The listing builds one solid part. Answer for the finished solid, in the listing's coordinates (mm). Face numbers are marked on the shaded views. A direction names the side the tool comes from. Give positions to 0.01 mm unless a question says otherwise; leave off trailing zeros. Loops run counter-clockwise (first coordinate to the right, second up) from the corner with the lowest first, then second, coordinate; pieces in that order, holes last. Notation, with made-up numbers: M -25.5,61.5 L -20.5,61.5 A16 ccw -20.5,69.5 Z; hole C -10,82.5 d3. An arc over 180 degrees is marked long. Return JSON: item names as keys, results as strings.
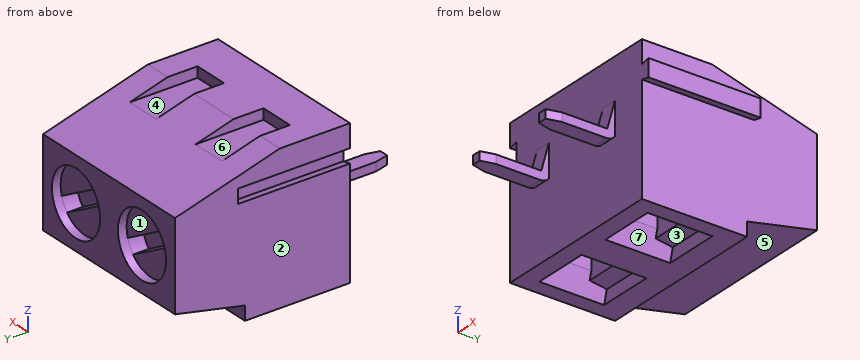
from build123d import *
from build123d.topology import SkipClean

# Parameters (mm, degrees)
BOSS_EXTRUDE1_DEPTH = 2.5
CUT_EXTRUDE1_DEPTH  = 1.25
CHAMFER1_SIZE       = 0.35
CHAMFER1_SIZE_2     = 1.3
CUT_EXTRUDE2_DEPTH  = 1
SKETCH5_R           = 1.825
CUT_EXTRUDE3_DEPTH  = 0.5
CUT_EXTRUDE4_DEPTH  = 0.9
BOSS_EXTRUDE3_DEPTH = 0.45
CHAMFER2_SIZE       = 0.2
CHAMFER2_SIZE2      = 0.79
MIRROR1_START       = -1.36978926
MIRROR1_OUTLINE_W   = 4
MIRROR1_OUTLINE_H   = 0.498489558
MIRROR1_DEPTH       = 0.193883275
LPATTERN1_COUNT     = 2
LPATTERN1_PITCH     = 5
BOSS_EXTRUDE2_DEPTH = 6.4
CUT_EXTRUDE5_DEPTH  = 6.4


# Read off the part's stored shape, not the designer's step: Mirror1
with BuildPart() as part:
    # Sketch2 → Boss-Extrude1 (new, symmetric)
    with BuildSketch(Plane(origin=(0, 0, 0), x_dir=(0, 0, -1), z_dir=(1, 0, 0))):
        Polygon((-4.15, 4), (-4.15, 0), (4.15, 0), (4.15, 6), (3.35, 6), (2.5, 9.99), (-2.5, 9.99), align=None)
    extrude(amount=BOSS_EXTRUDE1_DEPTH, both=True)

    # Sketch3 → Cut-Extrude1 (cut, symmetric)
    with BuildSketch(Plane(origin=(0, 0, 0), x_dir=(0, 0, -1), z_dir=(1, 0, 0))):
        Polygon((4.15, 1), (2.58, 1.84), (-2.25, 1.84), (-2.25, 3.7), (3.2988, 3.7), (3.4175, 4.7), (4.15, 4.7), align=None)
    extrude(amount=CUT_EXTRUDE1_DEPTH, both=True, mode=Mode.SUBTRACT)

    # Chamfer1
    # the kernel refuses this chamfer: 1.3, 0.35 mm, written as the material it takes off along each edge
    with BuildSketch(Plane(origin=(1.25, 4.7, -4.15), x_dir=(0.9905947308102195, 0, -0.1368286493795385), z_dir=(0, -1, 0))) as chamfer1_piece_1_section:
        Polygon((CHAMFER1_SIZE * 0.99059473081, CHAMFER1_SIZE * 0.13682864938), (-CHAMFER1_SIZE_2 * 0.13682864938, CHAMFER1_SIZE_2 * 0.99059473081), (0, 0), align=None)
    chamfer1_piece_1 = extrude(amount=7.075699234, mode=Mode.PRIVATE)
    chamfer1_piece_1 = split(chamfer1_piece_1, bisect_by=Plane(origin=(1.398374335, 1.802145787, -2.650751327), z_dir=(0, 0.8817303170442501, -0.47175380020201896)), keep=Keep.TOP, mode=Mode.PRIVATE)
    chamfer1_piece_1 = split(chamfer1_piece_1, bisect_by=Plane(origin=(1.398374335, 4.303686728, -3.370457615), z_dir=(0, -0.11787251100077023, -0.9930287363165143)), keep=Keep.TOP, mode=Mode.PRIVATE)
    add(chamfer1_piece_1, mode=Mode.SUBTRACT)
    with BuildSketch(Plane(origin=(1.25, 8.075699234, -4.15), x_dir=(0.9905947308102195, 0, -0.1368286493795385), z_dir=(0, -1, 0))) as chamfer1_piece_2_section:
        Polygon((CHAMFER1_SIZE * 0.99059473081, CHAMFER1_SIZE * 0.13682864938), (-CHAMFER1_SIZE_2 * 0.13682864938, CHAMFER1_SIZE_2 * 0.99059473081), (0, 0), align=None)
    chamfer1_piece_2 = extrude(amount=10.451398467, mode=Mode.PRIVATE)
    chamfer1_piece_2 = split(chamfer1_piece_2, bisect_by=Plane(origin=(1.281910217, 1.867643019, -2.528333882), z_dir=(0, 0.8817303170442501, -0.47175380020201896)), keep=Keep.TOP, mode=Mode.PRIVATE)
    chamfer1_piece_2 = split(chamfer1_piece_2, bisect_by=Plane(origin=(1.281910217, 3.7, -3.087047323), z_dir=(0, -1, 0)), keep=Keep.TOP, mode=Mode.PRIVATE)
    add(chamfer1_piece_2, mode=Mode.SUBTRACT)
    with BuildSketch(Plane(origin=(-1.25, 4.7, -4.15), x_dir=(-0.9905947308102195, 0, -0.1368286493795385), z_dir=(0, -1, 0))) as chamfer1_piece_3_section:
        Polygon((CHAMFER1_SIZE * 0.99059473081, -CHAMFER1_SIZE * 0.13682864938), (-CHAMFER1_SIZE_2 * 0.13682864938, -CHAMFER1_SIZE_2 * 0.99059473081), (0, 0), align=None)
    chamfer1_piece_3 = extrude(amount=7.075699234, mode=Mode.PRIVATE)
    chamfer1_piece_3 = split(chamfer1_piece_3, bisect_by=Plane(origin=(-1.398374335, 1.802145787, -2.650751327), z_dir=(0, 0.8817303170442501, -0.47175380020201896)), keep=Keep.TOP, mode=Mode.PRIVATE)
    chamfer1_piece_3 = split(chamfer1_piece_3, bisect_by=Plane(origin=(-1.398374335, 4.303686728, -3.370457615), z_dir=(0, -0.11787251100077023, -0.9930287363165143)), keep=Keep.TOP, mode=Mode.PRIVATE)
    add(chamfer1_piece_3, mode=Mode.SUBTRACT)
    with BuildSketch(Plane(origin=(-1.25, 8.075699234, -4.15), x_dir=(-0.9905947308102195, 0, -0.1368286493795385), z_dir=(0, -1, 0))) as chamfer1_piece_4_section:
        Polygon((CHAMFER1_SIZE * 0.99059473081, -CHAMFER1_SIZE * 0.13682864938), (-CHAMFER1_SIZE_2 * 0.13682864938, -CHAMFER1_SIZE_2 * 0.99059473081), (0, 0), align=None)
    chamfer1_piece_4 = extrude(amount=10.451398467, mode=Mode.PRIVATE)
    chamfer1_piece_4 = split(chamfer1_piece_4, bisect_by=Plane(origin=(-1.281910217, 1.867643019, -2.528333882), z_dir=(0, 0.8817303170442501, -0.47175380020201896)), keep=Keep.TOP, mode=Mode.PRIVATE)
    chamfer1_piece_4 = split(chamfer1_piece_4, bisect_by=Plane(origin=(-1.281910217, 3.7, -3.087047323), z_dir=(0, -1, 0)), keep=Keep.TOP, mode=Mode.PRIVATE)
    add(chamfer1_piece_4, mode=Mode.SUBTRACT)

    # Sketch4 → Cut-Extrude2 (cut, symmetric)
    with BuildSketch(Plane(origin=(0, 0, 0), x_dir=(0, 0, -1), z_dir=(1, 0, 0))):
        Polygon((-4.15, 2.3), (-3.55, 2.3), (-3.55, 6.178181818), (-4.15, 4), align=None)
    extrude(amount=CUT_EXTRUDE2_DEPTH, both=True, mode=Mode.SUBTRACT)

    # Sketch5 → Cut-Extrude3 (cut)
    with BuildSketch(Plane(origin=(0, 9.99, 0), x_dir=(1, 0, 0), z_dir=(0, 1, 0))):
        with Locations(Location((0, 0, 0), (0, 0, 270))):
            Circle(SKETCH5_R)
    extrude(amount=-CUT_EXTRUDE3_DEPTH, mode=Mode.SUBTRACT)

    # Sketch6 → Cut-Extrude4 (cut)
    with SkipClean():  # the faces are left unmerged after this step: merging them gives an invalid solid
        with BuildSketch(Plane(origin=(0, 9.49, 0), x_dir=(1, 0, 0), z_dir=(0, 1, 0))):
            with BuildLine():
                Line((-1.74206639, -0.543902284), (1.34206639, 1.236722607))
                ThreePointArc((1.34206639, 1.236722607), (1.580496362, 0.9125), (1.74206639, 0.543902284))
                Line((1.74206639, 0.543902284), (-1.34206639, -1.236722607))
                ThreePointArc((-1.34206639, -1.236722607), (-1.580496362, -0.9125), (-1.74206639, -0.543902284))
            make_face()
        extrude(amount=-CUT_EXTRUDE4_DEPTH, mode=Mode.SUBTRACT)

    # Sketch9 → Boss-Extrude3 (add, symmetric)
    with SkipClean():  # the faces are left unmerged after this step: merging them gives an invalid solid
        with BuildSketch(Plane(origin=(0, 0, 0), x_dir=(0, 0, -1), z_dir=(1, 0, 0))):
            with BuildLine():
                Line((0.25, -3.803865983), (-0.248489558, -3.803865983))
                Line((-0.248489558, -3.803865983), (-0.248489558, -0.432670696))
                Line((-0.248489558, -0.432670696), (-1.843660044, 0))
                Line((-1.843660044, 0), (0, 0))
                ThreePointArc((0, 0), (0.183674749, -0.206246517), (0.25, -0.474341649))
                Line((0.25, -0.474341649), (0.25, -3.803865983))
            make_face()
        extrude(amount=BOSS_EXTRUDE3_DEPTH, both=True)

    # Chamfer2
    chamfer2_edges = [part.edges().sort_by_distance(p)[0] for p in [
        (0.45, -3.803865983, -0.000755221),
    ]]
    chamfer2_side = [part.faces().sort_by_distance(p)[0] for p in [
        (0, -3.803865983, -0.000755221),
    ]]
    chamfer(chamfer2_edges, length=CHAMFER2_SIZE, length2=CHAMFER2_SIZE2, reference=chamfer2_side[0])

    # Mirror1 outline → Mirror1 (cut)
    with SkipClean():  # the faces are left unmerged after this step: merging them gives an invalid solid
        with BuildSketch(Plane(origin=(0, 0, 0), x_dir=(-0.2454218669703849, 0.9694163745330335, 0), z_dir=(0.9694163745330335, 0.2454218669703849, 0)).offset(MIRROR1_START)):
            with Locations((-3, -0.000755221)):
                Rectangle(MIRROR1_OUTLINE_W, MIRROR1_OUTLINE_H)
        extrude(amount=MIRROR1_DEPTH, mode=Mode.SUBTRACT)


with BuildPart() as lpattern1_1:
    # LPattern1: pattern copy
    add(part.part.moved(Location(Vector(-1, 0, 0) * (1 * LPATTERN1_PITCH))))


with BuildPart() as part_1:
    add(part.part)

    # Combine1: union LPattern1_1
    add(lpattern1_1.part)

    # Sketch8 → Boss-Extrude2 (add)
    with SkipClean():  # the faces are left unmerged after this step: merging them gives an invalid solid
        with BuildSketch(Plane.XZ):
            Polygon((3, 2.45), (2.5, 2.45), (2.5, 2.05), (3, 1.95), align=None)
            Polygon((3, 2.95), (2.5, 2.85), (2.5, 2.45), (3, 2.45), align=None)
        extrude(amount=-BOSS_EXTRUDE2_DEPTH)

    # Sketch8<3> → Cut-Extrude5 (cut)
    with SkipClean():  # the faces are left unmerged after this step: merging them gives an invalid solid
        with BuildSketch(Plane.XZ):
            Polygon((-7, 1.95), (-7, 2.95), (-7.5, 2.85), (-7.5, 2.05), align=None)
        extrude(amount=-CUT_EXTRUDE5_DEPTH, mode=Mode.SUBTRACT)


solid = part_1.part
(1) Given pin 1 (0.7 mm diameter, centred on x = 0.5, z = -1, fed in from +Y); pin 2 (0.6 mm diameter, centred on x = -7, z = 2.5, fed in from -Y); pin 3 (1 mm diameter, centred on x = -5, y = -2.5, fed in from +Z), each flat-ended and moving along its own axis, determine where each tip first touches the part or whether it passes through.
Values follow:
{"pin 1": "y = 9.49", "pin 2": "y = 0", "pin 3": "z = 0.25"}
(2) The part is cut by section A-A (y = -2.25). Determine the outline of the cut face in (x, z).
Values follow:
{"outline": "M -5.45,-0.25 L -4.55,-0.25 L -4.55,0.25 L -5.45,0.25 Z; M -0.45,-0.25 L 0.45,-0.25 L 0.45,0.25 L -0.45,0.25 Z"}
(3) The part is cut by section C-C (z = 1.5). Determine the outline of the cut face in (x, y), and give its area (3 significant figures).
Values follow:
{"outline": "M -7.5,0 L -5.45,0 L -5.45,-0.09 L -4.55,-0.09 L -4.55,0 L -0.45,0 L -0.45,-0.09 L 0.45,-0.09 L 0.45,0 L 2.5,0 L 2.5,9.99 L 1.04,9.99 L 1.04,9.49 L -1.04,9.49 L -1.04,9.99 L -3.96,9.99 L -3.96,9.49 L -6.04,9.49 L -6.04,9.99 L -7.5,9.99 Z; hole M -6.25,1.84 L -3.75,1.84 L -3.75,3.7 L -6.25,3.7 Z; hole M -1.25,1.84 L 1.25,1.84 L 1.25,3.7 L -1.25,3.7 Z", "area": "88.7 mm²"}
(4) Straight lines are drawn through the part: line 1 along X through (y, z) = (9.6, 0) (3 decimals); line 2 along Y through (x, z) = (-6, 1.75); line 3 along X through (y, z) = (6, -0.25). For each, find the intervals that lie inside material, in ascending order.
Values follow:
{"line 1": "-7.5 to -6.825, -3.175 to -1.825, 1.825 to 2.5", "line 2": "0 to 1.84, 3.7 to 9.99", "line 3": "-7.5 to 2.5"}
(5) The part is cut by section B-B (x = -3). Determine the outline of the cut face in (y, z), and give its area (3 significant figures).
Values follow:
{"outline": "M 0,-4.15 L 6,-4.15 L 6,-3.35 L 9.99,-2.5 L 9.99,2.5 L 4,4.15 L 0,4.15 Z", "area": "73.1 mm²"}
(6) A tool of negligible diameter and unlimited length cuts with its end or side. For the marked faces 1, 2, 3 and 4, from which of +Z, -Z, +X, -X, +Y, -Y can it reach the whole face along a straight path? Write none if from no direction.
Values follow:
{"face 1": "+Y", "face 2": "+Z, -Z, -X, +Y, -Y", "face 3": "-Z", "face 4": "+Z, +Y"}
(7) Determine the mould class of the marked faces 5, 6 and 7 for opening direction Y: released by +Y, released by -Y, zero draft, split by the parting line, or undercut.
Values follow:
{"face 5": "released by +Y", "face 6": "zero draft", "face 7": "undercut"}
(8) The part is cut by section D-D (y = 4.25). Determine the outline of the cut face in (x, z).
Values follow:
{"outline": "M -7.5,-4.15 L -6.6,-4.15 L -6.39,-3.36 L -3.61,-3.36 L -3.4,-4.15 L -1.6,-4.15 L -1.39,-3.36 L 1.39,-3.36 L 1.6,-4.15 L 2.5,-4.15 L 2.5,2.05 L 3,1.95 L 3,2.95 L 2.5,2.85 L 2.5,4.08 L 1,4.08 L 1,3.55 L -1,3.55 L -1,4.08 L -4,4.08 L -4,3.55 L -6,3.55 L -6,4.08 L -7.5,4.08 L -7.5,2.85 L -7,2.95 L -7,1.95 L -7.5,2.05 Z"}
